Here's how the part is built. I have some questions about the finished solid (model axes, mm). Face numbers are marked on the shaded views. A direction names the side the tool comes from. Round coordinates to 2 decimals unless told otherwise and drop trailing zeros. Order: outer loops, then holes, each group sorted by start corner. A loop starts at its lowest first (then second) coordinate and runs counter-clockwise, first axis right, second up.
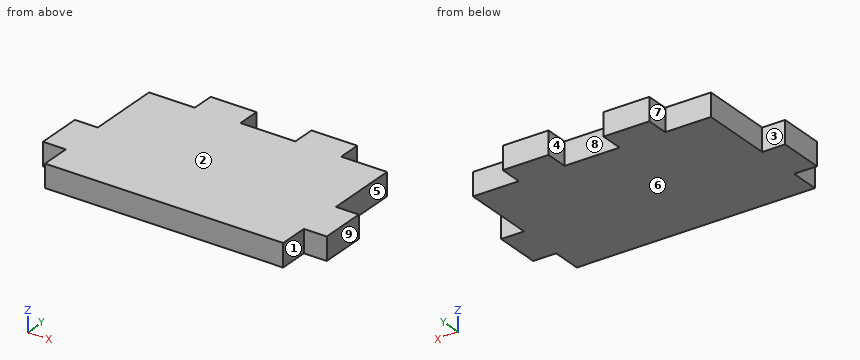
Autodesk Inventor part; units mm, degrees
ref_plane "YZ Plane" through (0, 0, 0) normal (1, 0, 0) x (0, 1, 0)
ref_plane "XZ Plane" through (0, 0, 0) normal (0, 1, 0) x (-1, 0, 0)
ref_plane "XY Plane" through (0, 0, 0) normal (0, 0, 1) x (1, 0, 0)
sketch "Sketch1" plane through (0, 0, 0) normal (0, 0, 1) x (1, 0, 0)
  line L0 (-18.7161, 14.4213) -> (-18.7161, -26.8537)
  line L1 (-18.7161, 14.4213) -> (47.3239, 14.4213)
  line L2 (47.3239, 14.4213) -> (47.3239, -26.8537)
  line L3 (47.3239, -26.8537) -> (-18.7161, -26.8537)
  line L4 (-18.7161, 14.4213) -> (-6.0161, 14.4213)
  line L5 (-6.0161, 14.4213) -> (-6.0161, 20.7713)
  line L6 (-6.0161, 20.7713) -> (6.6839, 20.7713)
  line L7 (6.6839, 20.7713) -> (6.6839, 14.4213)
  line L8 (47.3239, 14.4213) -> (34.6239, 14.4213)
  line L9 (34.6239, 14.4213) -> (34.6239, 20.7713)
  line L10 (34.6239, 20.7713) -> (21.9239, 20.7713)
  line L11 (21.9239, 20.7713) -> (21.9239, 14.4213)
  line L12 (-18.7161, 14.4213) -> (-18.7161, -5.8987)
  line L13 (-18.7161, -5.8987) -> (-25.0661, -5.8987)
  line L14 (-25.0661, -5.8987) -> (-25.0661, -18.5987)
  line L15 (-25.0661, -18.5987) -> (-18.7161, -18.5987)
  line L16 (47.3239, 14.4213) -> (47.3239, -5.8987)
  line L17 (47.3239, -5.8987) -> (53.6739, -5.8987)
  line L18 (53.6739, -5.8987) -> (53.6739, -18.5987)
  line L19 (53.6739, -18.5987) -> (47.3239, -18.5987)
  point P0 (0, 0)
  dimension "d0" = 41.275
  dimension "d1" = 66.04
  dimension "d2" = 12.7
  dimension "d3" = 6.35
  dimension "d4" = 12.7
  dimension "d5" = 12.7
  dimension "d6" = 12.7
  dimension "d7" = 20.32
  dimension "d8" = 6.35
  dimension "d9" = 12.7
  dimension "d10" = 20.32
  dimension "d11" = 6.35
extrude "Extrusion1" add sketch "Sketch1" along normal blind 6.35
properties part number "support 2"
1) If we section it at C-C (x = -11.5): Write out the boundary of the cut face in (y, z), plus the area to 3 significant figures.
2) We'd pull the mould along X, two halves only. Please class the marked faces 6, 7, 8 and 9: +X half, -X half, draft (parallel to the pull), parting line (faces both ways), or undercut.
3) I need wall thicknesses on line 1 (X direction, y = 16, z = 1.5); line 2 (Y direction, x = 8, z = 1); line 3 (X direction, y = 11, z = 1.75). Which ranges of each line are inside material? Lowest first, please.
4) For the marked faces 1, 2, 3, 4 and 5, which set-ups out of +Z, -Z, +X, -X, +Y, -Y let a thin tool reach every point of the face, with its end or its side?
5) If we section it at D-D (y = 2): Write out the boundary of the cut face in (x, z), plus the area to 3 significant figures.
6) I'm going to push flat-ended pins straight in: pin 1 (3 mm diameter, centred on x = -12, z = 3.5, fed in from +Y); pin 2 (1.9 mm diameter, centred on x = -22.5, z = 4, fed in from +Y); pin 3 (1 mm diameter, centred on y = 5, z = 2, fed in from -X). Where does each tip first touch, or does it pass through?
7) If we section it at B-B (z = 1.75): Write out the boundary of the cut face in (x, y).
8) If we section it at A-A (y = 16): Write out the boundary of the cut face in (x, z).
Solutions:
1. outline: (-26.85, 0) - (14.42, 0) - (14.42, 6.35) - (-26.85, 6.35) - close
1. area: 262 mm2
2. face 6: draft
2. face 7: -X half
2. face 8: undercut
2. face 9: +X half
3. line 1: x = -6.02 to 6.68, 21.92 to 34.62
3. line 2: y = -26.85 to 14.42
3. line 3: x = -18.72 to 47.32
4. face 1: +Z, -Z, +X, -Y
4. face 2: +Z, +X, -X, +Y, -Y
4. face 3: +Z, -Z, -X, +Y
4. face 4: +Z, -Z, +Y
4. face 5: +Z, -Z, +X, +Y
5. outline: (-18.72, 0) - (47.32, 0) - (47.32, 6.35) - (-18.72, 6.35) - close
5. area: 419 mm2
6. pin 1: stops at y = 14.42
6. pin 2: stops at y = -5.9
6. pin 3: stops at x = -18.72
7. outline: (-25.07, -18.6) - (-18.72, -18.6) - (-18.72, -26.85) - (47.32, -26.85) - (47.32, -18.6) - (53.67, -18.6) - (53.67, -5.9) - (47.32, -5.9) - (47.32, 14.42) - (34.62, 14.42) - (34.62, 20.77) - (21.92, 20.77) - (21.92, 14.42) - (6.68, 14.42) - (6.68, 20.77) - (-6.02, 20.77) - (-6.02, 14.42) - (-18.72, 14.42) - (-18.72, -5.9) - (-25.07, -5.9) - close
8. outline: (-6.02, 0) - (6.68, 0) - (6.68, 6.35) - (-6.02, 6.35) - close; (21.92, 0) - (34.62, 0) - (34.62, 6.35) - (21.92, 6.35) - close
